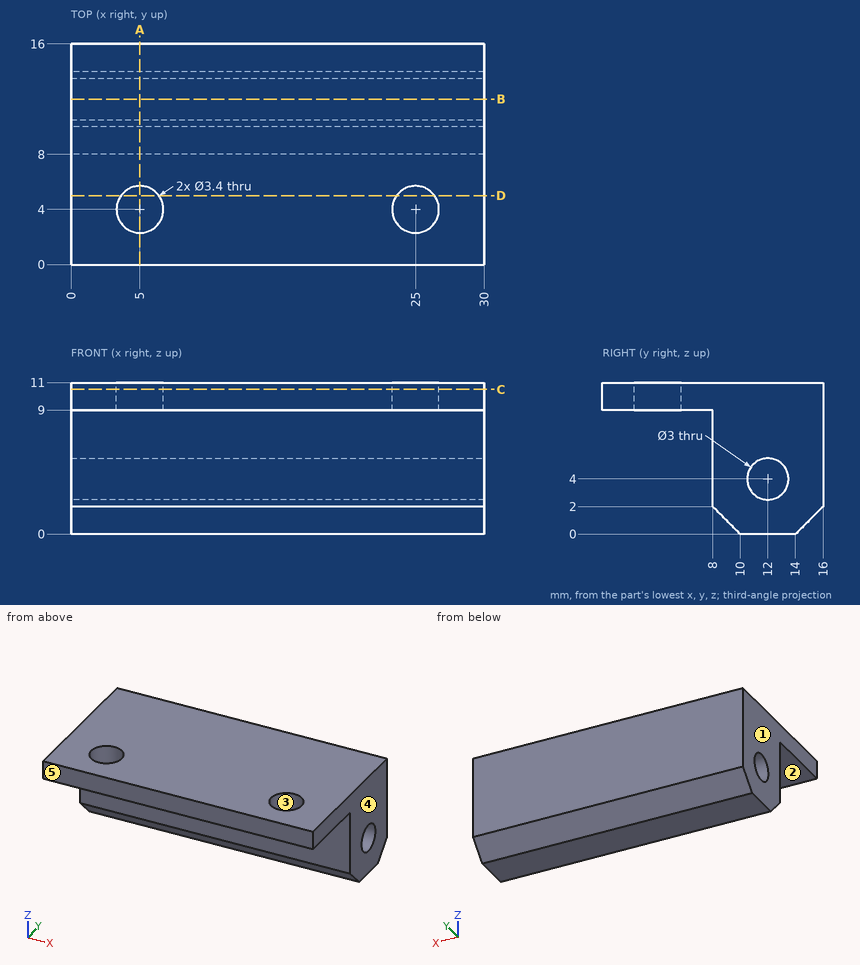
Here's the drawing with two shaded views (mm, measured from the low corner). I have some questions. A direction names the side the tool comes from. Give positions to 0.01 mm unless a question says otherwise; leave off trailing zeros. Order: outer loops, then holes, each group sorted by start corner. A loop starts at its lowest first (then second) coordinate and runs counter-clockwise, first axis right, second up. Notation, with made-up numbers: M 82,-34.75 L 109,-34.75 A11 ccw 109,-23.75 Z; hole C 45,54.25 d9. An arc over 180 degrees is marked long. One line per item, written item: value.
1) We'd pull the mould along X, two halves only. Please class the marked faces 3, 4 and 5: released by +X, released by -X, zero draft, split by the parting line, or undercut.
Answer sheet:
face 3: undercut
face 4: released by +X
face 5: zero draft
2) Please list where these lines run through material, in increasing order: line 1 along Y through (x, z) = (18.75, 4); line 2 along Y through (x, z) = (5, 9.8); line 3 along Z through (x, y) = (13.5, 5).
Answer sheet:
line 1: y = 8 to 10.5, 13.5 to 16
line 2: y = 0 to 2.3, 5.7 to 16
line 3: z = 9 to 11
3) I want a section at D-D, the plane y = 5. List the corners of the cut face in (x, z) for me.
Answer sheet:
outline: M 0,9 L 3.63,9 L 3.63,11 L 0,11 Z; M 6.37,9 L 23.63,9 L 23.63,11 L 6.37,11 Z; M 26.37,9 L 30,9 L 30,11 L 26.37,11 Z
4) I want a section at A-A, the plane x = 5. List the corners of the cut face in (y, z) for me, plus the area to 3 significant figures.
Answer sheet:
outline: M 0,9 L 2.3,9 L 2.3,11 L 0,11 Z; M 5.7,9 L 8,9 L 8,2 L 10,0 L 14,0 L 16,2 L 16,11 L 5.7,11 Z; hole C 12,4 d3
area: 86.1 mm^2
5) I want a section at C-C, the plane z = 10.5. List the corners of the cut face in (x, y) for me, plus the area to 3 significant figures.
Answer sheet:
outline: M 0,0 L 30,0 L 30,16 L 0,16 Z; hole C 5,4 d3.4; hole C 25,4 d3.4
area: 462 mm^2
6) On a 3-axis mill with a long thin cutter (end or side, diameter ignored), from which of +Z, -Z, +X, -X, +Y, -Y can I reach the whole of each face in a straight line? I mean the marked faces 1 and 2. Say none if no direction works.
Answer sheet:
face 1: +Z, -Z, -X, +Y, -Y
face 2: -Z, +X, -X, -Y
7) I want a section at B-B, the plane y = 12. List the corners of the cut face in (x, z) for me, plus the area to 3 significant figures.
Answer sheet:
outline: M 0,0 L 30,0 L 30,2.5 L 0,2.5 Z; M 0,5.5 L 30,5.5 L 30,11 L 0,11 Z
area: 240 mm^2
8) For P1, Ø2, axis at y = 5.5, z = 7, coming from the +X side; P2, Ø9, axis at x = 15.5, y = 5, coming from the -Z side; P3, Ø1, axis at x = 18.5, y = 4, coming from the -Z side; P4, Ø1, axis at x = 9.5, z = 4, coming from the -Y side, each with a flat end and sliding along its axis, tell me the tip position at first contact or that it passes through.
Answer sheet:
P1: passes through
P2: stops at z = 0.5
P3: stops at z = 9
P4: stops at y = 8
